Here's how the part is built. I have some questions about the finished solid (model axes, mm). A direction names the side the tool comes from. Coordinates: 2 decimals unless noted, no trailing zeros. Loops run counter-clockwise (first coordinate to the right, second up) from the corner with the lowest first, then second, coordinate; pieces in that order, holes last. Notation, with made-up numbers: (41.5, 52.5) -> (46.5, 52.5) arc R19 ccw to (46.5, 88.5) -> close; hole circle Ø9 at (-5.5, 55). An arc over 180 degrees is marked (long way). Answer as a JSON object with one key per item and string values. Group by question number.
Q1. I need wall thicknesses on line 1 (Y direction, x = -31.5, z = -5.75); line 2 (Y direction, x = 0, z = -1.25) (3 decimals). Which ranges of each line are inside material? Lowest first, please.
Q2. I want a section at B-B on z = -1.25. Count the separate pieces of the cut face and the enclosed holes in it, then the cut area to 3 significant figures.
Q3. On a 3-axis mill with a long thin cutter (end or side, diameter ignored), from which of +Z, -Z, +X, -X, +Y, -Y can I reach the whole of each face in a straight line? I mean faces 1 (the flat face through (-35, -25, -3)), 2 (the flat face through (35, -25, -3)), 3 (the flat face through (-20, 31.4, -3)), 4 (the flat face through (25, -35, -3)). Say none if no direction works.
Q4. Thinking about a two-plate mould opening in Y: for faces 5 (the flat face through (-15, -35, -3)), 6 (the flat face through (31.4, -20, -3)), 7 (the flat face through (-31.4, 20, -3)), 8 (the flat face through (0, -38, -3)), which applies, released by +Y, released by -Y, zero draft, split by the parting line, or undercut?
Q5. I want a section at A-A on y = -20.5. Write out the boundary of the cut face in (x, z).
Q6. I'm going to push flat-ended pins straight in: pin 1 (3.5 mm diameter, centred on x = -19, z = -3, fed in from +Y); pin 2 (3.5 mm diameter, centred on y = 19.5, z = -2.5, fed in from -X). Where does each tip first touch, or does it pass through?
```python
from build123d import *

# Parameters (mm, degrees)
F0_W     = 76
F0_H     = 76
F1_DEPTH = 6.6
F2_W     = 10
F2_H     = 6.6
F2_W_2   = 6.6
F2_H_2   = 10
F3_DEPTH = 6.6
F4_R     = 0.8
F5_DEPTH = 6.6


with BuildPart() as f1:
    # F0 (on Top) → F1 (new body)
    with BuildSketch(Plane.XY):
        Rectangle(F0_W, F0_H)
    extrude(amount=-F1_DEPTH)

    # F2 (on face) → F3 (cut, through all)
    with BuildSketch(Plane.XY):
        with Locations((20, 34.7)):
            Rectangle(F2_W, F2_H)
        with Locations((-20, 34.7)):
            Rectangle(F2_W, F2_H)
        with Locations((-34.7, -20)):
            Rectangle(F2_W_2, F2_H_2)
        with Locations((-34.7, 20)):
            Rectangle(F2_W_2, F2_H_2)
        with Locations((20, -34.7)):
            Rectangle(F2_W, F2_H)
        with Locations((-20, -34.7)):
            Rectangle(F2_W, F2_H)
        with Locations((34.7, 20)):
            Rectangle(F2_W_2, F2_H_2)
        with Locations((34.7, -20)):
            Rectangle(F2_W_2, F2_H_2)
    extrude(amount=-F3_DEPTH, mode=Mode.SUBTRACT)

    # F4 (on face) → F5 (cut, through all)
    with BuildSketch(Plane.XY):
        with Locations((0, 10.475)):
            Circle(F4_R)
        with Locations((0, -26.275)):
            Circle(F4_R)
    extrude(amount=-F5_DEPTH, mode=Mode.SUBTRACT)


solid = f1.part
```
Result set:
{
 "1": {"line 1": "y = -38 to -25, -15 to 15, 25 to 38", "line 2": "y = -38 to -27.075, -25.475 to 9.675, 11.275 to 38"},
 "2": {"separate pieces": "1", "enclosed holes": "2", "area": "5,240 mm²"},
 "3": {"face 1": "+Z, -Z, -X", "face 2": "+Z, -Z, +X", "face 3": "+Z, -Z, +Y", "face 4": "+Z, -Z, -Y"},
 "4": {"face 5": "zero draft", "face 6": "undercut", "face 7": "undercut", "face 8": "released by -Y"},
 "5": {"outline": "(-31.4, -6.6) -> (31.4, -6.6) -> (31.4, 0) -> (-31.4, 0) -> close"},
 "6": {"pin 1": "stops at y = 31.4", "pin 2": "stops at x = -31.4"}
}
